```python
from build123d import *

# Parameters (mm, degrees)
SKETCH1_W           = 200
SKETCH1_H           = 130
BOSS_EXTRUDE1_DEPTH = 3
SKETCH2_W           = 97
SKETCH2_H           = 70
CUT_EXTRUDE1_DEPTH  = 120.306328416
SKETCH3_W           = 3
SKETCH3_H           = 10
CUT_EXTRUDE2_DEPTH  = 120.306328416
LPATTERN1_COUNT     = 3
LPATTERN1_PITCH     = 20
SKETCH4_W           = 3
SKETCH4_H           = 10
CUT_EXTRUDE3_DEPTH  = 120.306328416
LPATTERN2_COUNT     = 7
LPATTERN2_PITCH     = 20
SKETCH5_W           = 3
SKETCH5_H           = 10
CUT_EXTRUDE4_DEPTH  = 120.306328416
LPATTERN3_COUNT     = 4
LPATTERN3_PITCH     = 20
SKETCH7_W           = 10
SKETCH7_H           = 3
CUT_EXTRUDE7_DEPTH  = 120.306328416
LPATTERN6_COUNT     = 5
LPATTERN6_PITCH     = 20
SKETCH8_W           = 10
SKETCH8_H           = 3
CUT_EXTRUDE8_DEPTH  = 120.306328416
LPATTERN8_COUNT     = 4
LPATTERN8_PITCH     = 20


with BuildPart() as part:
    # Sketch1 → Boss-Extrude1 (new body)
    with BuildSketch(Plane(origin=(0, 0, 0), x_dir=(1, 0, 0), z_dir=(0, 1, 0))):
        Rectangle(SKETCH1_W, SKETCH1_H)
    extrude(amount=BOSS_EXTRUDE1_DEPTH)

    # Sketch2 → Cut-Extrude1 (cut, through all)
    with BuildSketch(Plane(origin=(0, 3, 0), x_dir=(1, 0, 0), z_dir=(0, 1, 0))):
        with Locations((-51.5, 30)):
            Rectangle(SKETCH2_W, SKETCH2_H)
    extrude(amount=-CUT_EXTRUDE1_DEPTH, mode=Mode.SUBTRACT)

    # Sketch3 → Cut-Extrude2 (cut, through all)
    with BuildSketch(Plane(origin=(0, 3, 0), x_dir=(1, 0, 0), z_dir=(0, 1, 0))):
        with Locations((-98.5, -60)):
            Rectangle(SKETCH3_W, SKETCH3_H)
    cut_extrude2 = extrude(amount=-CUT_EXTRUDE2_DEPTH, mode=Mode.SUBTRACT)

    # LPattern1: Cut-Extrude2 ×3
    with Locations(*[(0, 0, -i * LPATTERN1_PITCH) for i in range(1, LPATTERN1_COUNT)]):
        add(cut_extrude2, mode=Mode.SUBTRACT)

    # Sketch4 → Cut-Extrude3 (cut, through all)
    with BuildSketch(Plane(origin=(0, 3, 0), x_dir=(1, 0, 0), z_dir=(0, 1, 0))):
        with Locations((98.5, -60)):
            Rectangle(SKETCH4_W, SKETCH4_H)
    cut_extrude3 = extrude(amount=-CUT_EXTRUDE3_DEPTH, mode=Mode.SUBTRACT)

    # LPattern2: Cut-Extrude3 ×7
    with Locations(*[(0, 0, -i * LPATTERN2_PITCH) for i in range(1, LPATTERN2_COUNT)]):
        add(cut_extrude3, mode=Mode.SUBTRACT)

    # Sketch5 → Cut-Extrude4 (cut, through all)
    with BuildSketch(Plane(origin=(0, 3, 0), x_dir=(1, 0, 0), z_dir=(0, 1, 0))):
        with Locations((-1.5, 60)):
            Rectangle(SKETCH5_W, SKETCH5_H)
    cut_extrude4 = extrude(amount=-CUT_EXTRUDE4_DEPTH, mode=Mode.SUBTRACT)

    # LPattern3: Cut-Extrude4 ×4
    with Locations(*[(0, 0, i * LPATTERN3_PITCH) for i in range(1, LPATTERN3_COUNT)]):
        add(cut_extrude4, mode=Mode.SUBTRACT)

    # Sketch7 → Cut-Extrude7 (cut, through all)
    with BuildSketch(Plane(origin=(0, 3, 0), x_dir=(1, 0, 0), z_dir=(0, 1, 0))):
        with Locations((-15, -6.5)):
            Rectangle(SKETCH7_W, SKETCH7_H)
    cut_extrude7 = extrude(amount=-CUT_EXTRUDE7_DEPTH, mode=Mode.SUBTRACT)

    # LPattern6: Cut-Extrude7 ×5
    with Locations(*[(-i * LPATTERN6_PITCH, 0, 0) for i in range(1, LPATTERN6_COUNT)]):
        add(cut_extrude7, mode=Mode.SUBTRACT)

    # Sketch8 → Cut-Extrude8 (cut, through all)
    with BuildSketch(Plane(origin=(0, 3, 0), x_dir=(1, 0, 0), z_dir=(0, 1, 0))):
        with Locations((78.5, 38.5)):
            Rectangle(SKETCH8_W, SKETCH8_H)
    cut_extrude8 = extrude(amount=-CUT_EXTRUDE8_DEPTH, mode=Mode.SUBTRACT)

    # LPattern8: Cut-Extrude8 ×4
    with Locations(*[(-i * LPATTERN8_PITCH, 0, 0) for i in range(1, LPATTERN8_COUNT)]):
        add(cut_extrude8, mode=Mode.SUBTRACT)


solid = part.part
```
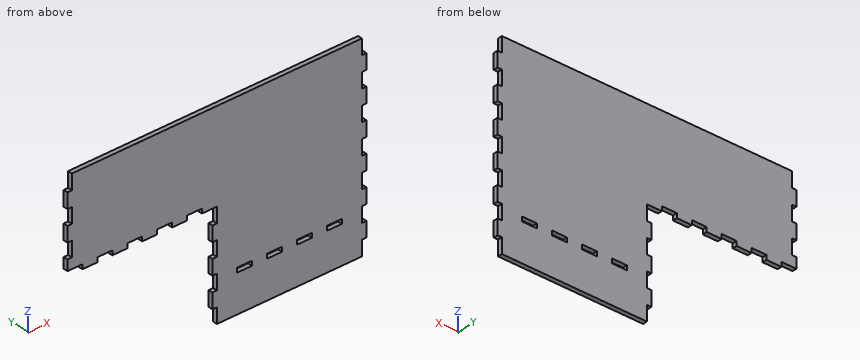
Could you check a few things on this model? Use its own coordinates, in mm. Round coordinates to 2 decimals unless told otherwise and drop trailing zeros. Loops run counter-clockwise (first coordinate to the right, second up) from the corner with the lowest first, then second, coordinate; pieces in that order, holes last.
Q1. I want a section at C-C (y = 0.75). Give the number of separate pieces and of enclosed holes in the cut face, and give its area (3 significant figures).
Q2. I want a section at D-D (x = -13). Write out the boundary of the cut face in (y, z), and give its area (3 significant figures).
Q3. I want a section at A-A (x = 59.5). Write out the boundary of the cut face in (y, z).
Q4. Please list where these lines run through material, in increasing order: L1, parallel to X at y = 0.7, z = -39; L2, parallel to Z at x = 21, y = 2.75; L3, parallel to X at y = 0.35, z = -59.
Q5. I want a section at B-B (z = 1). Write out the boundary of the cut face in (x, y), and give its area (3 significant figures).
Q6. For P1, Ø1.5, axis at y = 1, z = -38.5, coming from the -X side; P2, Ø1.5, axis at y = 1.5, z = -40.5, coming from the +X side; P3, Ø1.5, axis at y = 2, z = 61.5, coming from the -X side, each with a flat end and sliding along its axis, tell me the tip position at first contact or that it passes through.
Answer below:
1. separate pieces: 1
1. enclosed holes: 4
1. area: 18,500 mm2
2. outline: (0, 8) - (3, 8) - (3, 65) - (0, 65) - close
2. area: 171 mm2
3. outline: (0, -65) - (3, -65) - (3, -40) - (0, -40) - close; (0, -37) - (3, -37) - (3, 65) - (0, 65) - close
4. L1: x = 0 to 13.5, 23.5 to 33.5, 43.5 to 53.5, 63.5 to 73.5, 83.5 to 97
4. L2: z = -65 to -40, -37 to 65
4. L3: x = 0 to 97
5. outline: (0, 0) - (97, 0) - (97, 3) - (0, 3) - close
5. area: 291 mm2
6. P1: stops at x = 0
6. P2: stops at x = 97
6. P3: stops at x = -97
